Check sheet for the modelled part. Datum: model origin and axes. Units: mm. A direction names the side the tool comes from. Give positions to 0.01 mm unless a question says otherwise; leave off trailing zeros. Order: outer loops, then holes, each group sorted by start corner. A loop starts at its lowest first (then second) coordinate and runs counter-clockwise, first axis right, second up. Notation, with made-up numbers: (-15.75, 69.25) -> (3.25, 69.25) arc R22 cw to (3.25, 92.25) -> close; hole circle Ø2 at (3, 48). An arc over 180 degrees is marked (long way). Answer in a Markdown table with one row per item. Add a question column.
(1) Cross-section at D-D (x = 4). Record the cut outline in (y, z).
(2) Cross-section at C-C (z = 2). Record the cut outline in (x, y).
(3) Go/stop test with flat-tipped pins: pin 1 (12 mm diameter, centred on x = 30.5, y = 31, fed in from -Z); pin 2 (1 mm diameter, centred on x = 17.5, z = 1.5, fed in from +Y); pin 3 (1.2 mm diameter, centred on y = 33.5, z = 1, fed in from -X). Record where each tip stops, or that it passes through.
(4) Cross-section at B-B (x = 15). Record the cut outline in (y, z).
(5) Cross-section at A-A (y = 25.5). Record the cut outline in (x, z), then the cut area to 3 significant figures.
(6) Thickness scan on L1, parallel to X at y = -0.5, z = 1.3; L2, parallel to Y at x = 16.5, z = 1; L3, parallel to Y at x = 17, z = 1.55. Record the ranges inside material, lowest first. Write a range as [from, to].
(7) Set-up check for faces 4 (the face through (5.093, 50.726, 1.972)), 5 (the face through (33.228, 14.128, 1.972)), 6 (the face through (27, 5, 2)), 7 (the face through (-5, 23, 2)): record each of +Z, -Z, +X, -X, +Y, -Y from which the full face is reachable in a straight line by a thin tool's end or side.
(8) Release check for a two-part mould opening along X. For faces 1 (the face through (9.644, 25.927, 2.028)), 2 (the face through (-4, -3, 2)), 3 (the face through (11, 31, 0)) record: released by +X, released by -X, zero draft, split by the parting line, or undercut.
```python
from build123d import *

# Parameters (mm, degrees)
SKETCH1_R           = 2
BOSS_EXTRUDE1_DEPTH = 4
FILLET10_R          = 1
FILLET11_R          = 10
FILLET12_R          = 5
FILLET13_R          = 5
FILLET14_R          = 5
SKETCH2_R           = 2
CUT_EXTRUDE1_DEPTH  = 20


with BuildPart() as part:
    # Sketch1 → Boss-Extrude1 (new body)
    with BuildSketch(Plane.XY):
        with BuildLine():
            Line((-5, -5), (-5, 46.428571429))
            ThreePointArc((-5, 46.428571429), (5.360662074, 77.221028176), (35.086282243, 90.332329282))
            Line((35.086282243, 90.332329282), (35.086282243, 80.08008038))
            ThreePointArc((35.086282243, 80.08008038), (5.086282243, 50.08008038), (35.086282243, 20.08008038))
            Line((35.086282243, 20.08008038), (35.086282243, 14.08008038))
            ThreePointArc((35.086282243, 14.08008038), (31.017062028, 14.31079961), (27, 15))
            Line((27, 15), (27, -5))
            Line((27, -5), (-5, -5))
        make_face()
        Circle(SKETCH1_R, mode=Mode.SUBTRACT)
        with Locations((18, 0)):
            Circle(SKETCH1_R, mode=Mode.SUBTRACT)
    extrude(amount=BOSS_EXTRUDE1_DEPTH)

    # Fillet10
    fillet10_edges = [part.edges().sort_by_distance(p)[0] for p in [
        (35.086282243, 90.332329282, 2),
        (35.086282243, 80.08008038, 2),
        (35.086282243, 20.08008038, 2),
        (35.086282243, 14.08008038, 2),
    ]]
    fillet(fillet10_edges, radius=FILLET10_R)

    # Fillet11
    # the kernel refuses this fillet: 10 mm, written as the material it adds along each edge
    with BuildSketch(Plane(origin=(-5, 46.428571429, 0), x_dir=(-0.08596186737445177, 0.996298427860597, 0), z_dir=(0, 0, 1))) as fillet11_piece_1:
        with BuildLine():
            CenterArc((0.431926178, 9.999886119), FILLET11_R, 265.068661729, 4.657897264)
            Line((-0.427692496, 0.03690184), (0, 0))
            ThreePointArc((0, 0), (0.19210095, 0.000458397), (0.3842019, 0))
        make_face()
    extrude(amount=4)

    # Fillet12
    fillet12_edges = [part.edges().sort_by_distance(p)[0] for p in [
        (-5, -5, 2),
    ]]
    fillet(fillet12_edges, radius=FILLET12_R)

    # Fillet13
    fillet13_edges = [part.edges().sort_by_distance(p)[0] for p in [
        (27, -5, 2),
    ]]
    fillet(fillet13_edges, radius=FILLET13_R)

    # Fillet14
    fillet14_edges = [part.edges().sort_by_distance(p)[0] for p in [
        (27, 15, 2),
    ]]
    fillet(fillet14_edges, radius=FILLET14_R)

    # Sketch2 → Cut-Extrude1 (cut)
    with BuildSketch(Plane.XY.offset(4)):
        with Locations((10.086282243, 74.574977808)):
            Circle(SKETCH2_R)
        with Locations((11.117766586, 24.574977808)):
            Circle(SKETCH2_R)
    extrude(amount=-CUT_EXTRUDE1_DEPTH, mode=Mode.SUBTRACT)


solid = part.part
```
Answer below:
| question | item | result |
|---|---|---|
| 1 | outline | (-5, 0) -> (75.65, 0) -> (75.65, 4) -> (-5, 4) -> close |
| 2 | outline | (-5.03, 46.81) arc R10 cw to (-5, 46) -> (-5, 0) arc R5 ccw to (0, -5) -> (22, -5) arc R5 ccw to (27, 0) -> (27, 9.2) arc R5 cw to (32.38, 14.18) arc R36 ccw to (34.06, 14.09) arc R1 ccw to (35.09, 15.09) -> (35.09, 19.1) arc R1 ccw to (34.12, 20.1) arc R30 cw to (34.12, 80.06) arc R1 ccw to (35.09, 81.06) -> (35.09, 89.32) arc R1 ccw to (34.06, 90.32) arc R40.25 ccw to start; hole circle Ø4 at (0, 0); hole circle Ø4 at (10.09, 74.57); hole circle Ø4 at (11.12, 24.57); hole circle Ø4 at (18, 0) |
| 3 | pin 1 | passes through |
| 3 | pin 2 | stops at y = 86.53 |
| 3 | pin 3 | stops at x = -5 |
| 4 | outline | (-5, 0) -> (27.8, 0) -> (27.8, 4) -> (-5, 4) -> close; (72.36, 0) -> (84.96, 0) -> (84.96, 4) -> (72.36, 4) -> close |
| 5 | outline | (-5, 0) -> (9.34, 0) -> (9.34, 4) -> (-5, 4) -> close; (12.89, 0) -> (17.89, 0) -> (17.89, 4) -> (12.89, 4) -> close |
| 5 | area | 77.4 mm² |
| 6 | L1 | x = [-4.97, -1.94], [1.94, 16.06], [19.94, 26.97] |
| 6 | L2 | y = [-5, -1.32], [1.32, 26.53], [73.63, 85.78] |
| 6 | L3 | y = [-5, -1.73], [1.73, 26.15], [74.02, 86.04] |
| 7 | face 4 | +Z, -Z, +X |
| 7 | face 5 | +Z, -Z, -Y |
| 7 | face 6 | +Z, -Z, +X, -Y |
| 7 | face 7 | +Z, -Z, -X, -Y |
| 8 | face 1 | undercut |
| 8 | face 2 | released by -X |
| 8 | face 3 | zero draft |
